The model under review builds one solid part; all positions refer to its coordinate system, in mm. A direction names the side the tool comes from. Round coordinates to 2 decimals unless told otherwise and drop trailing zeros. Order: outer loops, then holes, each group sorted by start corner. A loop starts at its lowest first (then second) coordinate and runs counter-clockwise, first axis right, second up. Notation, with made-up numbers: M -17,10.5 L 32,10.5 A8 ccw 32,14.5 Z; hole C 35,81 d2. An arc over 180 degrees is marked long. Answer as a JSON object with one key per item and string values. Group by question number.
1. Add section C-C on y = -19. State the section outline as (x, z) points, and give its area (3 significant figures).
2. Mouldability with a two-part tool opening along Y and no side actions: class faces 1 (the face through (-6, -23, 3)), 2 (the face through (-11.715, 4.392, 0.301)), 3 (the face through (-5, 31, 6)) as released by +Y, released by -Y, zero draft, split by the parting line, or undercut.
3. Machinability: for faces 4 (the face through (5, 31, 6)), 5 (the face through (2.95, 10, 4)), 6 (the face through (0, 4, 0)), which of the approach directions +Z, -Z, +X, -X, +Y, -Y give a long, thin tool a straight path to every point of the face, cutting with its end or side? Answer none if there is none.
4. Clearance check with flat-ended pins moving along their axes: P1, Ø10.5, axis at x = 6.5, y = 1, coming from the +Z side; P2, Ø2, axis at x = 4, z = 6, coming from the +Y side. State where each tip first meets the part, or that it passes through.
5. Add section A-A on x = -7. State the section outline as (y, z) points.
6. To check wall thickness, follow probe 1 along X at (y, z) = (29.5, 4.25) (3 decimals); probe 2 along X at (y, z) = (17, 6.75) (3 decimals); probe 3 along Y at (x, z) = (6.25, 2.5). State the ranges of each line that lie inside material, in increasing order. Write a range as [from, to].
7. Add section D-D on x = -3.75. State the section outline as (y, z) points, and give its area (3 significant figures).
8. Add section B-B on z = 3.25. State the section outline as (x, y) points (3 decimals).
```python
from build123d import *

# Parameters (mm, degrees)
SKETCH1_W           = 24
SKETCH1_H           = 58
BOSS_EXTRUDE1_DEPTH = 2
BOSS_EXTRUDE2_DEPTH = 2.5
CUT_EXTRUDE3_DEPTH  = 3
CUT_EXTRUDE4_DEPTH  = 3
SKETCH7_W           = 3.525
SKETCH7_H           = 40.926519782
BOSS_EXTRUDE3_DEPTH = 5
FILLET1_R           = 1


with BuildPart() as part:
    # Sketch1 → Boss-Extrude1 (new body)
    with BuildSketch(Plane.XY):
        with Locations((0, 4)):
            Rectangle(SKETCH1_W, SKETCH1_H)
    extrude(amount=BOSS_EXTRUDE1_DEPTH)

    # Sketch2 → Boss-Extrude2 (add)
    with BuildSketch(Plane.XY.offset(2)):
        Polygon((12, 33), (-12, 33), (-12, -25), (12, -25), (12, 9), align=None)
        Polygon((-10, -23), (-10, 23), (-10, 31), (10, 31), (10, 23), (10, -23), align=None, mode=Mode.SUBTRACT)
    extrude(amount=BOSS_EXTRUDE2_DEPTH)

    # Sketch5 → Cut-Extrude3 (cut, through all)
    with BuildSketch(Plane.XZ.offset(-31)):
        with BuildLine():
            Line((-2.95, 4.5), (2.95, 4.5))
            ThreePointArc((2.95, 4.5), (0, 1.55), (-2.95, 4.5))
        make_face()
    extrude(amount=-CUT_EXTRUDE3_DEPTH, mode=Mode.SUBTRACT)

    # Sketch6 → Cut-Extrude4 (cut, through all)
    with BuildSketch(Plane(origin=(0, -23, 0), x_dir=(1, 0, 0), z_dir=(0, 1, 0))):
        with BuildLine():
            Line((-2.5, -4.5), (2.5, -4.5))
            ThreePointArc((2.5, -4.5), (0, -2), (-2.5, -4.5))
        make_face()
    extrude(amount=-CUT_EXTRUDE4_DEPTH, mode=Mode.SUBTRACT)

    # Sketch7 → Boss-Extrude3 (add)
    with BuildSketch(Plane.XY.offset(2)):
        with Locations((-4.7125, 10.536740109)):
            Rectangle(SKETCH7_W, SKETCH7_H)
        with Locations((4.7125, 10.536740109)):
            Rectangle(SKETCH7_W, SKETCH7_H)
    extrude(amount=BOSS_EXTRUDE3_DEPTH)

    # Fillet1
    fillet1_edges = [part.edges().sort_by_distance(p)[0] for p in [
        (0, -25, 0),
        (-12, 4, 0),
        (0, 33, 0),
        (12, 4, 0),
        (12, -25, 2.25),
        (-12, -25, 2.25),
        (-12, 33, 2.25),
        (12, 33, 2.25),
    ]]
    fillet(fillet1_edges, radius=FILLET1_R)


solid = part.part
```
Recorded:
{
 "1": {"outline": "M -12,1 A1 ccw -11,0 L 11,0 A1 ccw 12,1 L 12,4.5 L 10,4.5 L 10,2 L -10,2 L -10,4.5 L -12,4.5 Z", "area": "57.6 mm²"},
 "2": {"face 1": "undercut", "face 2": "zero draft", "face 3": "released by +Y"},
 "3": {"face 4": "+Z, +X, -X, +Y", "face 5": "+Z", "face 6": "-Z, +X, -X, +Y, -Y"},
 "4": {"P1": "stops at z = 7", "P2": "stops at y = 31"},
 "5": {"outline": "M -25,1 A1 ccw -24,0 L 32,0 A1 ccw 33,1 L 33,4.5 L 31,4.5 L 31,2 L -23,2 L -23,4.5 L -25,4.5 Z"},
 "6": {"probe 1": "x = [-12, -10], [-6.475, -2.95], [2.95, 6.475], [10, 12]", "probe 2": "x = [-6.475, -2.95], [2.95, 6.475]", "probe 3": "y = [-25, -23], [-9.93, 33]"},
 "7": {"outline": "M -25,1 A1 ccw -24,0 L 32,0 A1 ccw 33,1 L 33,4.5 L 31,4.5 L 31,7 L -9.93,7 L -9.93,2 L -23,2 L -23,4.5 L -25,4.5 Z", "area": "330 mm²"},
 "8": {"outline": "M -12,-24 A1 ccw -11,-25 L -2.165,-25 L -2.165,-23 L -10,-23 L -10,31 L -6.475,31 L -6.475,-9.927 L -2.95,-9.927 L -2.95,31 L -2.672,31 L -2.672,33 L -11,33 A1 ccw -12,32 Z; M 2.165,-25 L 11,-25 A1 ccw 12,-24 L 12,32 A1 ccw 11,33 L 2.672,33 L 2.672,31 L 2.95,31 L 2.95,-9.927 L 6.475,-9.927 L 6.475,31 L 10,31 L 10,-23 L 2.165,-23 Z"}
}
